Design review of the part built by this model. Coordinates are the model's own, in mm. Face numbers are marked on the shaded views. A direction names the side the tool comes from. Give positions to 0.01 mm unless a question says otherwise; leave off trailing zeros. Write each loop counter-clockwise with the first axis right and the second up, starting at its lowest first coordinate (ties: lowest second). Pieces come first, ordered by that corner, then holes. Notation, with made-up numbers: (10, 2.25) -> (61, 2.25) arc R25 cw to (61, 24.25) -> close; hole circle Ø4 at (-15.75, -28.75). An arc over 180 degrees is marked (long way). Write each question's results on one line, items separated by ' | '. Start each with the question number.
(1) Clearance check with flat-ended pins moving along their axes: pin 1 (1.6 mm diameter, centred on x = 163.5, y = 1.5, fed in from +Z); pin 2 (3 mm diameter, centred on x = 36, y = -6.5, fed in from -Z); pin 3 (7.5 mm diameter, centred on y = -5.5, z = -24.5, fed in from +X). State where each tip first meets the part, or that it passes through.
(2) For the marked faces 1 and 2, list the 3-axis set-ups (+Z, -Z, +X, -X, +Y, -Y) from which the entire face can be reached by the end or side of a thin tool; tool diameter is ignored.
(3) Take a section at B-B (z = -31.5). State the section outline as (x, y) points, plus the area to 3 significant figures.
(4) Take a section at D-D (x = 138). State the section outline as (y, z) points.
(5) Take a section at A-A (x = 34.85). State the section outline as (y, z) points (3 decimals), plus the area to 3 significant figures.
(6) Take a section at C-C (z = -68.5). State the section outline as (x, y) points, plus the area to 3 significant figures.
(7) Mouldability with a two-part tool opening along X and no side actions: class the marked faces 3, 4 and 5 as released by +X, released by -X, zero draft, split by the parting line, or undercut.
(8) To check wall thickness, follow probe 1 along X at (y, z) = (1.35, -86.5) (3 decimals); probe 2 along Z at (x, y) = (83.92, 0.5) (3 decimals); probe 3 along X at (y, z) = (-8.5, -9). State the ranges of each line that lie inside material, in increasing order.
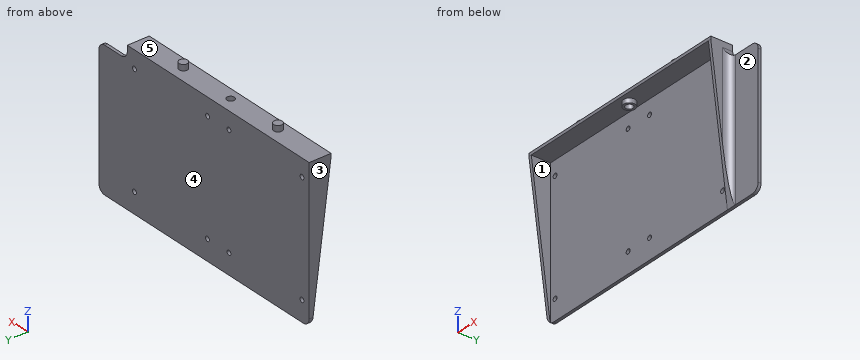
from build123d import *

# Parameters (mm, degrees)
SKETCH1_W           = 10
SKETCH1_H           = 100.5
SKETCH1_R           = 1.625
SKETCH1_W_2         = 69.85
BOSS_EXTRUDE1_DEPTH = 2
SKETCH3_W           = 149.7
SKETCH3_H           = 2
BOSS_EXTRUDE2_DEPTH = 2
SKETCH4_W           = 100.5
SKETCH4_H           = 2
BOSS_EXTRUDE3_DEPTH = 2
BOSS_EXTRUDE4_DEPTH = 2
SKETCH6_W           = 8
SKETCH6_H           = 15
BOSS_EXTRUDE5_DEPTH = 3
CUT_EXTRUDE1_DEPTH  = 10
FILLET1_R           = 3
CUT_EXTRUDE2_DEPTH  = 10
BOSS_EXTRUDE6_START = 3
SKETCH10_R          = 4
SKETCH10_R_2        = 2.55
BOSS_EXTRUDE6_DEPTH = 3
SKETCH12_R          = 2.875
BOSS_EXTRUDE7_DEPTH = 4
SKETCH13_W          = 10.946886228
SKETCH13_H          = 17.580383234
SKETCH13_W_2        = 10.296538922
SKETCH13_H_2        = 23.433508982
CUT_EXTRUDE3_DEPTH  = 43
SKETCH15_W          = 24
SKETCH15_H          = 93.5
BOSS_EXTRUDE8_DEPTH = 2
FILLET2_R           = 5
FILLET3_R           = 5


with BuildPart() as part:
    # Sketch1 → Boss-Extrude1 (new body)
    # profile 1 of 3: a face of its own
    with BuildSketch(Plane(origin=(0, 0, 0), x_dir=(1, 0, 0), z_dir=(0, 1, 0))):
        with Locations((74.85, 50.25)):
            Rectangle(SKETCH1_W, SKETCH1_H)
    # profile 2 of 3: a face of its own
    with BuildSketch(Plane(origin=(0, 0, 0), x_dir=(1, 0, 0), z_dir=(0, 1, 0))):
        Polygon((0, 0), (69.85, 0), (69.85, 100.5), (0, 100.5), (0, 86.5), align=None)
        with Locations(Location((4.07, 9.9, 0), (0, 0, 270))):
            Circle(SKETCH1_R, mode=Mode.SUBTRACT)
        with BuildLine():
            ThreePointArc((64.165, 9.9), (64.640951481, 11.049048519), (65.79, 11.525))
            ThreePointArc((65.79, 11.525), (66.939048519, 11.049048519), (67.415, 9.9))
            ThreePointArc((67.415, 9.9), (65.79, 8.275), (64.165, 9.9))
        make_face(mode=Mode.SUBTRACT)
        with BuildLine():
            ThreePointArc((5.695, 86.5), (4.07, 84.875), (2.445, 86.5))
            ThreePointArc((2.445, 86.5), (4.07, 88.125), (5.695, 86.5))
        make_face(mode=Mode.SUBTRACT)
        with BuildLine():
            ThreePointArc((65.79, 84.875), (64.640951481, 85.350951481), (64.165, 86.5))
            ThreePointArc((64.165, 86.5), (65.79, 88.125), (67.415, 86.5))
            ThreePointArc((67.415, 86.5), (66.939048519, 85.350951481), (65.79, 84.875))
        make_face(mode=Mode.SUBTRACT)
    # profile 3 of 3: a face of its own
    with BuildSketch(Plane(origin=(0, 0, 0), x_dir=(1, 0, 0), z_dir=(0, 1, 0))):
        with Locations((114.775, 50.25)):
            Rectangle(SKETCH1_W_2, SKETCH1_H)
        with Locations(Location((83.92, 9.9, 0), (0, 0, 270))):
            Circle(SKETCH1_R, mode=Mode.SUBTRACT)
        with Locations(Location((145.64, 9.9, 0), (0, 0, 270))):
            Circle(SKETCH1_R, mode=Mode.SUBTRACT)
        with Locations(Location((83.92, 86.5, 0), (0, 0, 270))):
            Circle(SKETCH1_R, mode=Mode.SUBTRACT)
        with Locations(Location((145.64, 86.5, 0), (0, 0, 270))):
            Circle(SKETCH1_R, mode=Mode.SUBTRACT)
    extrude(amount=BOSS_EXTRUDE1_DEPTH)

    # Sketch3 → Boss-Extrude2 (add)
    with BuildSketch(Plane.XY):
        Polygon((-10, 2), (-10, -13), (159.7, -13), (159.7, 2), (149.7, 2), (149.7, 0), (0, 0), (0, 2), align=None)
        with Locations((74.85, 1)):
            Rectangle(SKETCH3_W, SKETCH3_H)
    extrude(amount=BOSS_EXTRUDE2_DEPTH)

    # Sketch4 → Boss-Extrude3 (add)
    with BuildSketch(Plane.ZY):
        Polygon((0, 0), (-100.5, 0), (0, -13), align=None)
        with Locations((-50.25, 1)):
            Rectangle(SKETCH4_W, SKETCH4_H)
    extrude(amount=BOSS_EXTRUDE3_DEPTH)

    # Sketch5 → Boss-Extrude4 (add)
    with BuildSketch(Plane(origin=(149.7, 0, 0), x_dir=(0, 0, -1), z_dir=(1, 0, 0))):
        Polygon((100.5, 0), (0, -13), (0, 2), (100.5, 2), align=None)
    extrude(amount=BOSS_EXTRUDE4_DEPTH)

    # Sketch6 → Boss-Extrude5 (add)
    with BuildSketch(Plane(origin=(0, 0, 0), x_dir=(-1, 0, 0), z_dir=(0, 0, -1))):
        with Locations((6, -5.5)):
            Rectangle(SKETCH6_W, SKETCH6_H)
        with Locations((-155.7, -5.5)):
            Rectangle(SKETCH6_W, SKETCH6_H)
    extrude(amount=BOSS_EXTRUDE5_DEPTH)

    # Sketch8 → Cut-Extrude1 (cut)
    with BuildSketch(Plane(origin=(0, 0, -3), x_dir=(-1, 0, 0), z_dir=(0, 0, -1))):
        with BuildLine():
            ThreePointArc((-153.15, -5.5), (-155.7, -2.95), (-158.25, -5.5))
            Line((-158.25, -5.5), (-153.15, -5.5))
        make_face()
        with BuildLine():
            Line((-153.15, -5.5), (-158.25, -5.5))
            ThreePointArc((-158.25, -5.5), (-155.7, -8.05), (-153.15, -5.5))
        make_face()
        with BuildLine():
            ThreePointArc((3.45, -5.5), (6, -8.05), (8.55, -5.5))
            Line((8.55, -5.5), (3.45, -5.5))
        make_face()
        with BuildLine():
            Line((3.45, -5.5), (8.55, -5.5))
            ThreePointArc((8.55, -5.5), (6, -2.95), (3.45, -5.5))
        make_face()
    extrude(amount=-CUT_EXTRUDE1_DEPTH, mode=Mode.SUBTRACT)

    # Fillet1
    fillet1_edges = [part.edges().sort_by_distance(p)[0] for p in [
        (159.7, 2, -0.5),
        (-10, 2, -0.5),
        (-10, -13, -0.5),
        (159.7, -13, -0.5),
    ]]
    fillet(fillet1_edges, radius=FILLET1_R)

    # Sketch9 → Cut-Extrude2 (cut)
    with BuildSketch(Plane(origin=(0, 0, 0), x_dir=(-1, 0, 0), z_dir=(0, 0, -1))):
        with BuildLine():
            ThreePointArc((-72.3, -6.5), (-73.046877708, -4.696877708), (-74.85, -3.95))
            Line((-74.85, -3.95), (-74.85, -9.05))
            ThreePointArc((-74.85, -9.05), (-73.046877708, -8.303122292), (-72.3, -6.5))
        make_face()
        with BuildLine():
            Line((-74.85, -9.05), (-74.85, -3.95))
            ThreePointArc((-74.85, -3.95), (-77.4, -6.5), (-74.85, -9.05))
        make_face()
    extrude(amount=-CUT_EXTRUDE2_DEPTH, mode=Mode.SUBTRACT)

    # Sketch10 → Boss-Extrude6 (add)
    with BuildSketch(Plane(origin=(0, 0, 0), x_dir=(-1, 0, 0), z_dir=(0, 0, -1)).offset(BOSS_EXTRUDE6_START)):
        with Locations(Location((-74.85, -6.5, 0), (0, 0, 180))):
            Circle(SKETCH10_R)
        with Locations((-74.85, -6.5)):
            Circle(SKETCH10_R_2, mode=Mode.SUBTRACT)
    extrude(amount=-BOSS_EXTRUDE6_DEPTH)

    # Sketch12 → Boss-Extrude7 (add)
    with BuildSketch(Plane.XY.offset(2)):
        with Locations((34.85, -6.5)):
            Circle(SKETCH12_R)
        with Locations((114.85, -6.5)):
            Circle(SKETCH12_R)
    extrude(amount=BOSS_EXTRUDE7_DEPTH)

    # Sketch13 → Cut-Extrude3 (cut)
    with BuildSketch(Plane(origin=(0, 0, -3), x_dir=(-1, 0, 0), z_dir=(0, 0, -1))):
        with Locations((-157.173443114, -6.790191617)):
            Rectangle(SKETCH13_W, SKETCH13_H)
        with Locations((7.148269461, -9.716754491)):
            Rectangle(SKETCH13_W_2, SKETCH13_H_2)
    extrude(amount=-CUT_EXTRUDE3_DEPTH, mode=Mode.SUBTRACT)

    # Sketch15 → Boss-Extrude8 (add)
    with BuildSketch(Plane(origin=(0, 2, 0), x_dir=(1, 0, 0), z_dir=(0, 1, 0))):
        with Locations((163.7, 53.75)):
            Rectangle(SKETCH15_W, SKETCH15_H)
    extrude(amount=-BOSS_EXTRUDE8_DEPTH)

    # Fillet2
    # the kernel refuses this fillet: 5 mm, written as the material it adds along each edge
    with BuildSketch(Plane(origin=(151.7, 2, -7), x_dir=(1, 0, 0), z_dir=(0, -1, 0))) as fillet2_piece_1:
        with BuildLine():
            CenterArc((FILLET2_R, FILLET2_R), FILLET2_R, 180, 90)
            Line((0, FILLET2_R), (0, 0))
            Line((0, 0), (FILLET2_R, 0))
        make_face()
    extrude(amount=2)
    # the kernel refuses this fillet: 5 mm, written as the material it takes off along each edge
    with BuildSketch(Plane(origin=(175.7, 14.5, -100.5), x_dir=(-1, 0, 0), z_dir=(0, -1, 0)), Plane(origin=(175.7, 14.5, -7), x_dir=(0, 0, -1), z_dir=(0, -1, 0))) as fillet2_2_piece_1:
        with BuildLine():
            CenterArc((FILLET2_R, -FILLET2_R), FILLET2_R, 90, 90)
            Line((0, -FILLET2_R), (0, 0))
            Line((0, 0), (FILLET2_R, 0))
        make_face()
    extrude(amount=27, mode=Mode.SUBTRACT)
    with BuildSketch(Plane(origin=(-2, 14.5, -100.5), x_dir=(1, 0, 0), z_dir=(0, -1, 0))) as fillet2_2_piece_2:
        with BuildLine():
            CenterArc((FILLET2_R, FILLET2_R), FILLET2_R, 180, 90)
            Line((0, FILLET2_R), (0, 0))
            Line((0, 0), (FILLET2_R, 0))
        make_face()
    extrude(amount=27, mode=Mode.SUBTRACT)

    # Fillet3
    fillet3_edges = [part.edges().sort_by_distance(p)[0] for p in [
        (151.7, 0, -51.25),
    ]]
    fillet(fillet3_edges, radius=FILLET3_R)


solid = part.part
Report:
1) pin 1: z = -7 | pin 2: z = 0 | pin 3: x = 152.9
2) face 1: -Z, -Y | face 2: +Z, -Z, +X, -Y
3) outline: (-2, -8.93) -> (0, -8.93) -> (0, 0) -> (149.7, 0) -> (149.7, -8.93) -> (151.7, -8.93) -> (151.7, -5) arc R5 cw to (156.7, 0) -> (175.7, 0) -> (175.7, 2) -> (-2, 2) -> close | area: 396 mm2
4) outline: (-13, 0) -> (0, 0) -> (0, -100.5) -> (2, -100.5) -> (2, 2) -> (-13, 2) -> close
5) outline: (-13, 0) -> (0, 0) -> (0, -100.5) -> (2, -100.5) -> (2, 2) -> (-3.625, 2) -> (-3.625, 6) -> (-9.375, 6) -> (-9.375, 2) -> (-13, 2) -> close | area: 254 mm2
6) outline: (-2, -4.14) -> (0, -4.14) -> (0, 0) -> (149.7, 0) -> (149.7, -4.14) -> (151.77, -4.14) arc R5 cw to (156.7, 0) -> (175.7, 0) -> (175.7, 2) -> (-2, 2) -> close | area: 377 mm2
7) face 3: released by -X | face 4: zero draft | face 5: undercut
8) probe 1: -2 to 2.445, 5.695 to 64.165, 67.415 to 82.295, 85.545 to 144.015, 147.265 to 175.7 | probe 2: -100.5 to -88.125, -84.875 to -11.525, -8.275 to 2 | probe 3: -2 to 0, 149.7 to 151.7
